For this review, take the finished solid that the model builds, in its own axes (mm). A direction names the side the tool comes from. Give positions to 0.01 mm unless a question says otherwise; leave off trailing zeros. Write each loop counter-clockwise with the first axis right and the second up, starting at its lowest first coordinate (ties: lowest second). Pieces come first, ordered by that corner, then holes. Notation, with made-up numbers: M 65,-8.5 L 112,-8.5 A22 ccw 112,12.5 Z; hole C 71,83.5 d10. An arc over 180 degrees is marked long. Write item = value, one per line.
```python
from build123d import *

# Parameters (mm, degrees)
EXTRUDE001_DEPTH  = 51
ARRAY002_Y_COUNT  = 9
ARRAY002_Y_PITCH  = 15
CYLINDER003_R     = 2.1
CYLINDER003_DEPTH = 102
ARRAY001_Y_COUNT  = 2
ARRAY001_Y_PITCH  = 157
ARRAY001_Z_COUNT  = 2
ARRAY001_Z_PITCH  = 30
BOX004_W          = 3
BOX004_H          = 180
BOX004_DEPTH      = 60


with BuildPart() as side_vent_array:
    # Sketch001 → Extrude001 (new body, symmetric)
    with BuildSketch(Plane.YZ):
        with BuildLine():
            Line((-3, 50), (-3, 10))
            ThreePointArc((-3, 10), (0, 7), (3, 10))
            Line((3, 50), (3, 10))
            ThreePointArc((3, 50), (0, 53), (-3, 50))
        make_face()
    extrude(amount=EXTRUDE001_DEPTH, both=True)

    # Array002 Y: side vent array ×9


with BuildPart() as side_vent_array_1:
    add(side_vent_array.part)
    with Locations(*[(0, i * ARRAY002_Y_PITCH, 0) for i in range(1, ARRAY002_Y_COUNT)]):
        add(side_vent_array.part)


with BuildPart() as side_vent_array_2:
    # Array002 placement: moved
    add(side_vent_array_1.part.moved(Location((0, 30, 0))))


with BuildPart() as side_hole_fusion:
    # Cylinder003 → Cylinder003 (new body)
    with BuildSketch(Plane(origin=(-51, 13, 15), x_dir=(0, 0, -1), z_dir=(1, 0, 0))):
        Circle(CYLINDER003_R)
    extrude(amount=CYLINDER003_DEPTH)

    # Array001 Y: side hole fusion ×2


with BuildPart() as side_hole_fusion_1:
    add(side_hole_fusion.part)
    with Locations(*[(0, i * ARRAY001_Y_PITCH, 0) for i in range(1, ARRAY001_Y_COUNT)]):
        add(side_hole_fusion.part)

    # Array001 Z: side hole fusion ×2


with BuildPart() as side_hole_fusion_2:
    add(side_hole_fusion_1.part)
    with Locations(*[(0, 0, i * ARRAY001_Z_PITCH) for i in range(1, ARRAY001_Z_COUNT)]):
        add(side_hole_fusion_1.part)

    # Fusion001: union side vent array
    add(side_vent_array_2.part)


with BuildPart() as psu_side_cut001:
    # Box004 → Box004 (new body)
    with BuildSketch(Plane(origin=(48, 3, 0), x_dir=(1, 0, 0), z_dir=(0, 0, 1))):
        with Locations((1.5, 90)):
            Rectangle(BOX004_W, BOX004_H)
    extrude(amount=BOX004_DEPTH)

    # Cut001: cut side hole fusion
    add(side_hole_fusion_2.part, mode=Mode.SUBTRACT)


solid = psu_side_cut001.part
```
1. We need section B-B, the plane y = 75. Write out the cut boundary in (x, z), then the cut area to 3 significant figures.
Responses:
outline = M 48,0 L 51,0 L 51,7 L 48,7 Z; M 48,53 L 51,53 L 51,60 L 48,60 Z
area = 42.0 mm2
2. We need section C-C, the plane z = 15. Count the separate pieces of the cut face and the enclosed holes in it, then the cut area to 3 significant figures.
Responses:
separate_pieces = 12
enclosed_holes = 0
area = 353 mm2
3. Machinability: for faces 1 (the face through (49, 94, 0)), 2 (the face through (50, 63, 30)), which of the approach directions +Z, -Z, +X, -X, +Y, -Y give a long, thin tool a straight path to every point of the face, cutting with its end or side? Answer none if there is none.
Responses:
face_1 = -Z, +X, -X, +Y, -Y
face_2 = +X, -X
4. We need section A-A, the plane y = 170. Write out the cut boundary in (x, z), then the cut area to 3 significant figures.
Responses:
outline = M 48,0 L 51,0 L 51,12.9 L 48,12.9 Z; M 48,17.1 L 51,17.1 L 51,42.9 L 48,42.9 Z; M 48,47.1 L 51,47.1 L 51,60 L 48,60 Z
area = 155 mm2
5. For line 1 along Z through (x, y) = (50.2, 170); line 2 along Z through (x, y) = (49.55, 44), list the stretches that pass through material, from the lowest coordinate up. Write a range as from..to.
Responses:
line_1 = 0..12.9, 17.1..42.9, 47.1..60
line_2 = 0..7.17, 52.83..60
6. The part is to be moulded in two halves that separate along Y. For faces 3 (the face through (49, 94, 60)), 4 (the face through (50, 135, 7)), say which applies: +Y half, -Y half, draft (parallel to the pull), parting line (faces both ways), or undercut.
Responses:
face_3 = draft
face_4 = undercut
